The model under review builds one solid part; all positions refer to its coordinate system, in mm. A direction names the side the tool comes from. Coordinates: 2 decimals unless noted, no trailing zeros. Write each loop counter-clockwise with the first axis right and the second up, starting at its lowest first coordinate (ties: lowest second). Pieces come first, ordered by that corner, then holes. Notation, with made-up numbers: (6, -23) - (17, -23) arc R17 ccw to (17, -10) - close; hole circle Ø2 at (14, 53). An arc over 180 degrees is marked (long way). Return JSON: item names as keys, results as strings. Group by question number.
(1) We need section B-B on x = 6.5. State the section outline as (y, z) points (3 decimals), then the cut area to 3 significant figures.
(2) For pin 1 Ø8 at (y, z) = (-1, 2) entering from +X; pin 2 Ø1 at (x, y) = (2.5, -1) entering from +Z; pin 3 Ø1 at (x, z) = (8, 2) entering from +Y, all flat-tipped, find the tip position at first contact; note any pin that passes through.
(3) To check wall thickness, follow L1, parallel to X at y = 3.5, z = 6.5; L2, parallel to Y at x = 7.25, z = 1.25; L3, parallel to Z at x = 3, y = 2.75. State the ranges of each line that lie inside material, in increasing order. Write a range as from..to.
(4) Tool access review of faces 5 (the face through (4.93, -5.307, 3.007)), 6 (the face through (0, -5, 4)), 7 (the face through (4.93, 5.307, -3.007)): name each direction out of +Z, -Z, +X, -X, +Y, -Y from which nothing blocks a thin tool from reaching the whole face with its end or side.
(5) We need section A-A on y = 0. State the section outline as (x, z) points (3 decimals), then the cut area to 3 significant figures.
(6) We need section C-C on z = -1. State the section outline as (x, y) points.
(7) We need section D-D on z = -4. State the section outline as (x, y) points.
(8) Draft analysis for pull direction Z (two halves, no side actions). For faces 1 (the face through (-0.99, 7.81, -1.73)), 2 (the face through (4.1, 3.3, -0.7)), 3 (the face through (-2, -2, 3)), 4 (the face through (5, 0, 6.1)), state which applies: released by +Z, released by -Z, zero draft, split by the parting line, or undercut.
Autodesk Inventor part; units mm, degrees
ref_plane "YZ Plane" through (0, 0, 0) normal (1, 0, 0) x (0, 1, 0)
ref_plane "XZ Plane" through (0, 0, 0) normal (0, 1, 0) x (-1, 0, 0)
ref_plane "XY Plane" through (0, 0, 0) normal (0, 0, 1) x (1, 0, 0)
sketch "Sketch1" plane through (0, 0, 0) normal (1, 0, 0) x (0, 1, 0)
  line L0 (0, 0) -> (0, 6.1) construction
  line L1 (3.5218, 6.1) -> (7.0437, 0)
  line L2 (7.0437, 0) -> (3.5218, -6.1)
  line L3 (3.5218, -6.1) -> (-3.5218, -6.1)
  line L4 (-3.5218, -6.1) -> (-7.0437, 0)
  line L5 (-7.0437, 0) -> (-3.5218, 6.1)
  line L6 (-3.5218, 6.1) -> (3.5218, 6.1)
  dimension "d0" = 6.1
extrude "Extrusion1" add sketch "Sketch1" along normal blind 10
sketch "Sketch2" plane through (0, 0, 0) normal (-1, 0, 0) x (0, 0, 1)
  circle A0 centre (0, 0) radius 3.375
  circle A1 centre (0, 0) radius 8
  dimension "d3" = 6.75
  dimension "d4" = 16
extrude "Extrusion2" add sketch "Sketch2" along normal blind 2
sketch "Sketch3" plane through (0, 0, 0) normal (-1, 0, 0) x (0, 0, 1)
  circle A0 centre (0, 0) radius 3.375
extrude "Extrusion3" cut sketch "Sketch3" against normal blind 10
properties part number "smallHub 9-28"
Ans:
{
 "1": {"outline": "(-7.044, 0) - (-3.522, -6.1) - (3.522, -6.1) - (7.044, 0) - (3.522, 6.1) - (-3.522, 6.1) - close; hole circle Ø6.75 at (0, 0)", "area": "93.1 mm²"},
 "2": {"pin 1": "x = 10", "pin 2": "z = 6.1", "pin 3": "y = 6.18"},
 "3": {"L1": "-2..0", "L2": "-6.32..-3.13, 3.13..6.32", "L3": "-6.1..-1.96, 1.96..6.1"},
 "4": {"face 5": "+Z, +X, -Y", "face 6": "+X", "face 7": "-Z, +X, +Y"},
 "5": {"outline": "(-2, -8) - (0, -8) - (0, -6.1) - (10, -6.1) - (10, -3.375) - (-2, -3.375) - close; (-2, 3.375) - (10, 3.375) - (10, 6.1) - (0, 6.1) - (0, 8) - (-2, 8) - close", "area": "73.0 mm²"},
 "6": {"outline": "(-2, -7.94) - (0, -7.94) - (0, -6.47) - (10, -6.47) - (10, -3.22) - (-2, -3.22) - close; (-2, 3.22) - (10, 3.22) - (10, 6.47) - (0, 6.47) - (0, 7.94) - (-2, 7.94) - close"},
 "7": {"outline": "(-2, -6.93) - (0, -6.93) - (0, -4.73) - (10, -4.73) - (10, 4.73) - (0, 4.73) - (0, 6.93) - (-2, 6.93) - close"},
 "8": {"face 1": "split by the parting line", "face 2": "undercut", "face 3": "zero draft", "face 4": "released by +Z"}
}
